from build123d import *

# Parameters (mm, degrees)
EXTRUDE_THIN1_DEPTH = 50
SKETCH3_R           = 30
BOSS_EXTRUDE1_DEPTH = 50
SKETCH4_R           = 20
CUT_EXTRUDE1_DEPTH  = 110.083453206


with BuildPart() as part:
    # Sketch1 → Extrude-Thin1 (new body, symmetric)
    with BuildSketch(Plane.XY):
        Polygon((-50, 0), (50, 0), (111.28355545, -51.423008775), (104.855679353, -59.083453206), (46.360297657, -10), (-50, -10), align=None)
    extrude(amount=EXTRUDE_THIN1_DEPTH, both=True)

    # Sketch3 → Boss-Extrude1 (add)
    with BuildSketch(Plane(origin=(0, 0, 0), x_dir=(1, 0, 0), z_dir=(0, 1, 0))):
        Circle(SKETCH3_R)
    extrude(amount=BOSS_EXTRUDE1_DEPTH)

    # Sketch4 → Cut-Extrude1 (cut, through all)
    with BuildSketch(Plane(origin=(0, 50, 0), x_dir=(1, 0, 0), z_dir=(0, 1, 0))):
        Circle(SKETCH4_R)
    extrude(amount=-CUT_EXTRUDE1_DEPTH, mode=Mode.SUBTRACT)


solid = part.part
The model under review builds one solid part; all positions refer to its coordinate system, in mm. A direction names the side the tool comes from. Round coordinates to 2 decimals unless told otherwise and drop trailing zeros. Order: outer loops, then holes, each group sorted by start corner. A loop starts at its lowest first (then second) coordinate and runs counter-clockwise, first axis right, second up. Notation, with made-up numbers: (-5, -7) -> (4, -7) arc R15 ccw to (4, 2) -> close; hole circle Ø10 at (57, 35). An arc over 180 degrees is marked (long way). Write item = value, one per line. Start each with the question number.
Item 1: Clearance check with flat-ended pins moving along their axes: pin 1 Ø5 at (x, y) = (0.5, 14) entering from +Z; pin 2 Ø2 at (y, z) = (-14.5, 6) entering from -X; pin 3 Ø6 at (y, z) = (16, -5) entering from +X. State where each tip first meets the part, or that it passes through.
Item 2: Mouldability with a two-part tool opening along X and no side actions: class faces 4 (the face through (108.115, -55.2, 0.7)), 5 (the face through (-4.336, 20.42, 19.524)), 6 (the face through (-29.97, 24.65, -1.32)) as released by +X, released by -X, zero draft, split by the parting line, or undercut.
Item 3: For line 1 along Z through (x, y) = (0, 14.5); line 2 along X through (y, z) = (32, -11), list the stretches that pass through material, from the lowest coordinate up.
Item 4: Consider section C-C on y = 17. Write out the cut boundary in (x, z), plus the area to 3 significant figures.
Item 5: Consider section B-B on z = 0. Write out the cut boundary in (x, y), plus the area to 3 significant figures.
Item 6: Consider section D-D on z = -34.5. Write out the cut boundary in (x, y), plus the area to 3 significant figures.
Item 7: For faces 1 (the face through (-50, -5, 1)), 2 (the face through (-23, -10, 1)), 3 (the face through (-23, 0, 23)), list the 3-axis set-ups (+Z, -Z, +X, -X, +Y, -Y) from which the entire face can be reached by the end or side of a thin tool; tool diameter is ignored.
Item 8: Consider section A-A on x = 0. Write out the cut boundary in (y, z), plus the area to 3 significant figures.
Conclusion:
q1.pin_1 = 30
q1.pin_2 = 50.53
q1.pin_3 = 29.93
q2.face_4 = released by +X
q2.face_5 = undercut
q2.face_6 = split by the parting line
q3.line_1 = -30 to -20, 20 to 30
q3.line_2 = -27.91 to -16.7, 16.7 to 27.91
q4.outline = circle Ø60 at (0, 0); hole circle Ø40 at (0, 0)
q4.area = 1,570 mm2
q5.outline = (-50, -10) -> (-20, -10) -> (-20, 50) -> (-30, 50) -> (-30, 0) -> (-50, 0) -> close; (20, -10) -> (46.36, -10) -> (104.86, -59.08) -> (111.28, -51.42) -> (50, 0) -> (30, 0) -> (30, 50) -> (20, 50) -> close
q5.area = 2,360 mm2
q6.outline = (-50, -10) -> (46.36, -10) -> (104.86, -59.08) -> (111.28, -51.42) -> (50, 0) -> (-50, 0) -> close
q6.area = 1,760 mm2
q7.face_1 = +Z, -Z, -X, +Y, -Y
q7.face_2 = +Z, -Z, -X, -Y
q7.face_3 = +Y
q8.outline = (-10, -50) -> (0, -50) -> (0, -30) -> (50, -30) -> (50, -20) -> (-10, -20) -> close; (-10, 20) -> (50, 20) -> (50, 30) -> (0, 30) -> (0, 50) -> (-10, 50) -> close
q8.area = 1,600 mm2
